Work out the finished part from the listing and answer in its coordinate system (mm). A direction names the side the tool comes from. Give positions to 0.01 mm unless a question says otherwise; leave off trailing zeros. Order: outer loops, then holes, each group sorted by start corner. A loop starts at its lowest first (then second) coordinate and runs counter-clockwise, first axis right, second up.
Autodesk Inventor part; units mm, degrees
ref_plane "YZ Plane" through (0, 0, 0) normal (1, 0, 0) x (0, 1, 0)
ref_plane "XZ Plane" through (0, 0, 0) normal (0, 1, 0) x (-1, 0, 0)
ref_plane "XY Plane" through (0, 0, 0) normal (0, 0, 1) x (1, 0, 0)
sketch "Sketch1" plane through (0, 0, 0) normal (0, 0, 1) x (1, 0, 0)
  circle A0 centre (0, 0) radius 12.5 construction
  circle A1 centre (0, -8.5) radius 1.5 construction
  circle A2 centre (0, 8.5) radius 1.5 construction
  line L0 (-29, -17.5) -> (49, -17.5)
  line L1 (49, -17.5) -> (49, 12.5)
  line L2 (49, 12.5) -> (-29, 12.5)
  line L3 (-29, 12.5) -> (-29, -17.5)
  line L4 (-29, 12.5) -> (-19, 12.5)
  line L5 (-19, 12.5) -> (-19, 15.5)
  line L6 (-19, 15.5) -> (-29, 15.5)
  line L7 (-29, 15.5) -> (-29, 12.5)
  line L8 (10, 12.5) -> (27.5, 12.5)
  line L9 (19, 12.5) -> (29, 12.5)
  line L10 (29, 12.5) -> (29, 15.5)
  line L11 (29, 15.5) -> (19, 15.5)
  line L12 (19, 15.5) -> (19, 12.5)
  line L13 (12.5, 2.5) -> (15.5, 2.5)
  line L14 (15.5, 2.5) -> (15.5, -7.5)
  line L15 (15.5, -7.5) -> (12.5, -7.5)
  line L16 (12.5, -7.5) -> (12.5, 2.5)
  circle A3 centre (0, 0) radius 4
  circle A4 centre (0, -8.5) radius 1.5
  circle A5 centre (0, 8.5) radius 1.5
  point P0 (15.5, -2.5)
  point P1 (49, -2.5)
  dimension "d0" = 25
  dimension "d1" = 3
  dimension "d2" = 3
  dimension "d3" = 17
  dimension "d4" = 8.5
  dimension "d5" = 10
  dimension "d6" = 3
  dimension "d10" = 29
  dimension "d11" = 10
  dimension "d12" = 3
  dimension "d13" = 48
  dimension "d14" = 20
  dimension "d15" = 30
  dimension "d16" = 3
  dimension "d17" = 10
  dimension "d20" = 8
  dimension "d21" = 3
extrude "Extrusion1" add sketch "Sketch1" along normal blind 3
equation "\"d13\" = 2 * d10 - d11"
equation "\"d21\" = d1"
properties part number "Motor mount plate"
1. The part is cut by section B-B (z = 2). Write down the section's boundary in (x, y).
Findings below:
outline: (-29, -17.5) - (49, -17.5) - (49, 12.5) - (29, 12.5) - (29, 15.5) - (19, 15.5) - (19, 12.5) - (-19, 12.5) - (-19, 15.5) - (-29, 15.5) - close; hole circle Ø8 at (0, 0); hole circle Ø3 at (0, -8.5); hole circle Ø3 at (0, 8.5); hole (12.5, -7.5) - (15.5, -7.5) - (15.5, 2.5) - (12.5, 2.5) - close
2. Which of the six approach directions +Z, -Z, +X, -X, +Y, -Y give full straight-line access (tool end or side, diameter ignored) to faces 4 (the face through (29, 14, 1)), 5 (the face through (49, -3, 1)), 6 (the face through (9, -1, 0)), 7 (the face through (15.5, -2, 1)), 8 (the face through (-19, 14, 1))?
Findings below:
face 4: +Z, -Z, +X, +Y
face 5: +Z, -Z, +X, +Y, -Y
face 6: -Z, +X, -X, +Y, -Y
face 7: +Z, -Z
face 8: +Z, -Z, +Y
3. Straight lines are drawn through the part: probe 1 along Y at (x, z) = (0, 0.9); probe 2 along X at (y, z) = (-3, 1.35); probe 3 along X at (y, z) = (1, 2.3). For each, find the intervals that lie inside material, in ascending order.
Findings below:
probe 1: y = -17.5 to -10, -7 to -4, 4 to 7, 10 to 12.5
probe 2: x = -29 to -2.65, 2.65 to 12.5, 15.5 to 49
probe 3: x = -29 to -3.87, 3.87 to 12.5, 15.5 to 49
4. Given P1, Ø1.5, axis at x = 40, z = 2, coming from the +Y side; P2, Ø3, axis at x = -6.5, y = -2.5, coming from the -Z side, each flat-ended and moving along its own axis, determine where each tip first touches the part or whether it passes through.
Findings below:
P1: stops at y = 12.5
P2: stops at z = 0
5. The part is cut by section D-D (y = 0). Write down the section's boundary in (x, z), then the cut area to 3 significant figures.
Findings below:
outline: (-29, 0) - (-4, 0) - (-4, 3) - (-29, 3) - close; (4, 0) - (12.5, 0) - (12.5, 3) - (4, 3) - close; (15.5, 0) - (49, 0) - (49, 3) - (15.5, 3) - close
area: 201 mm2
6. The part is cut by section C-C (x = 0). Write down the section's boundary in (y, z).
Findings below:
outline: (-17.5, 0) - (-10, 0) - (-10, 3) - (-17.5, 3) - close; (-7, 0) - (-4, 0) - (-4, 3) - (-7, 3) - close; (4, 0) - (7, 0) - (7, 3) - (4, 3) - close; (10, 0) - (12.5, 0) - (12.5, 3) - (10, 3) - close
7. The mould has two halves that part along X. Classify faces 1 (the face through (-29, -1, 1)), 2 (the face through (14, -7.5, 1)), 3 (the face through (9, -1, 3)): pulls with the +X half, pulls with the -X half, needs draft (parallel to the pull), parting line crosses it, or undercut.
Findings below:
face 1: pulls with the -X half
face 2: undercut
face 3: needs draft
8. The part is cut by section A-A (y = 8.5). Write down the section's boundary in (x, z).
Findings below:
outline: (-29, 0) - (-1.5, 0) - (-1.5, 3) - (-29, 3) - close; (1.5, 0) - (49, 0) - (49, 3) - (1.5, 3) - close
